```python
from build123d import *

# Parameters (mm, degrees)
SKETCH2_OUTSIDE_W  = 79.82
SKETCH2_OUTSIDE_H  = 79.82
SKETCH2_OUTSIDE_R  = 1.6
CUT_EXTRUDE1_DEPTH = 10
SKETCH3_R          = 12
CUT_EXTRUDE2_DEPTH = 10


with BuildPart() as part:
    # Sketch1 → Revolve1 (revolve)
    with BuildSketch(Plane.XY, mode=Mode.PRIVATE) as revolve1_sk:
        Polygon((0, 0), (0, 13.335), (10.67, 13.335), (10.67, 30), (13.06, 30), (13.06, 14.095), (19.18, 14.095), (19.18, 11.90625), (27.18, 11.90625), (27.18, 0), align=None)
    revolve(revolve1_sk.sketch.rotate(Axis((0, 0, 0), (1, 0, 0)), 90), axis=Axis((0, 0, 0), (1, 0, 0)))  # turned: the seam where the file's is

    # Sketch2 outside → Cut-Extrude1 (cut)
    with BuildSketch(Plane.ZY.offset(-10.67)):
        Rectangle(SKETCH2_OUTSIDE_W, SKETCH2_OUTSIDE_H)
        with BuildLine():
            Line((-14.225, 18.225), (14.225, 18.225))
            ThreePointArc((14.225, 18.225), (17.053427125, 17.053427125), (18.225, 14.225))
            Line((18.225, 14.225), (18.225, -14.225))
            ThreePointArc((18.225, -14.225), (17.053427125, -17.053427125), (14.225, -18.225))
            Line((14.225, -18.225), (-14.225, -18.225))
            ThreePointArc((-14.225, -18.225), (-17.053427125, -17.053427125), (-18.225, -14.225))
            Line((-18.225, -14.225), (-18.225, 14.225))
            ThreePointArc((-18.225, 14.225), (-17.053427125, 17.053427125), (-14.225, 18.225))
        make_face(mode=Mode.SUBTRACT)
        with Locations((-14.29, 14.29)):
            Circle(SKETCH2_OUTSIDE_R)
        with Locations((14.29, 14.29)):
            Circle(SKETCH2_OUTSIDE_R)
        with Locations((14.29, -14.29)):
            Circle(SKETCH2_OUTSIDE_R)
        with Locations((-14.29, -14.29)):
            Circle(SKETCH2_OUTSIDE_R)
    extrude(amount=-CUT_EXTRUDE1_DEPTH, mode=Mode.SUBTRACT)

    # Sketch3 → Cut-Extrude2 (cut)
    with BuildSketch(Plane.ZY):
        Circle(SKETCH3_R)
    extrude(amount=-CUT_EXTRUDE2_DEPTH, mode=Mode.SUBTRACT)


solid = part.part
```
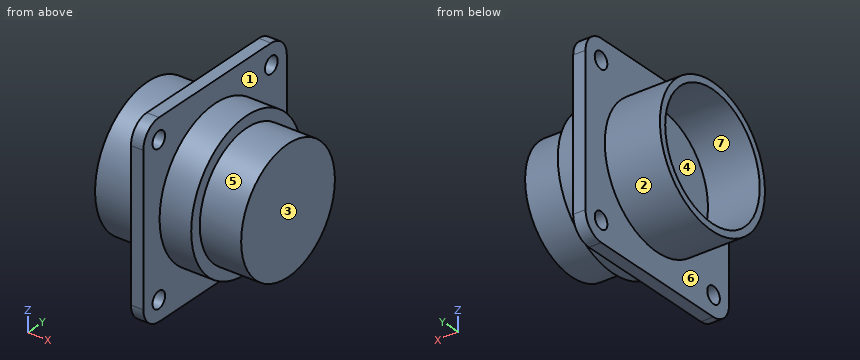
Can you work these out from the model? Positions are in its coordinate system, mm. Face numbers are marked on the shaded views. A direction names the side the tool comes from. Round coordinates to 2 decimals unless told otherwise and drop trailing zeros. Order: outer loops, then holes, each group sorted by start corner. A loop starts at its lowest first (then second) coordinate and runs counter-clockwise, first axis right, second up.
(1) If we section it at D-D (z = 15): Please give me the cut outline in (x, y).
Results are:
outline: (10.67, -18.15) - (13.06, -18.15) - (13.06, -15.72) - (10.67, -15.72) - close; (10.67, -12.86) - (13.06, -12.86) - (13.06, 12.86) - (10.67, 12.86) - close; (10.67, 15.72) - (13.06, 15.72) - (13.06, 18.15) - (10.67, 18.15) - close
(2) I'm going to push flat-ended pins straight in: pin 1 (10 mm diameter, centred on x = 22.5, y = -6.5, fed in from -Z); pin 2 (4 mm diameter, centred on x = 21, z = -3.5, fed in from +Y); pin 3 (3.5 mm diameter, centred on y = 14.29, z = 14.29, fed in from +X); pin 4 (1.9 mm diameter, centred on y = -14.29, z = 14.29, fed in from +X). Where does each tip first touch, or does it pass through?
Results are:
pin 1: stops at z = -13.82
pin 2: stops at y = 13.84
pin 3: stops at x = 13.06
pin 4: passes through
(3) If I drill on L1, parallel to Y at x = 11.8, z = -14.29; L2, parallel to X at y = -10, z = 0.5; L3, parallel to Z at x = 8.25, y = -11, over which ranges is the centre line in solid material (lowest first)?
Results are:
L1: y = -18.22 to -15.89, -12.69 to 12.69, 15.89 to 18.22
L2: x = 10 to 27.18
L3: z = -7.54 to -4.8, 4.8 to 7.54
(4) If we section it at A-A (x = 12.5): Please give me the cut outline in (y, z) (3 decimals).
Results are:
outline: (-18.225, -14.225) arc R4 ccw to (-14.225, -18.225) - (14.225, -18.225) arc R4 ccw to (18.225, -14.225) - (18.225, 14.225) arc R4 ccw to (14.225, 18.225) - (-14.225, 18.225) arc R4 ccw to (-18.225, 14.225) - close; hole circle Ø3.2 at (-14.29, -14.29); hole circle Ø3.2 at (-14.29, 14.29); hole circle Ø3.2 at (14.29, -14.29); hole circle Ø3.2 at (14.29, 14.29)
(5) On a 3-axis mill with a long thin cutter (end or side, diameter ignored), from which of +Z, -Z, +X, -X, +Y, -Y can I reach the whole of each face in a straight line? I mean the marked faces 1, 2 and 3. Say none if no direction works.
Results are:
face 1: +X
face 2: -X
face 3: +Z, -Z, +X, +Y, -Y
(6) We'd pull the mould along Y, two halves only. Please class the marked faces 4, 5, 6 and 7: +Y half, -Y half, draft (parallel to the pull), parting line (faces both ways), or undercut.
Results are:
face 4: undercut
face 5: parting line
face 6: draft
face 7: undercut
(7) If we section it at B-B (y = 0): Please give me the cut outline in (x, z) (3 decimals).
Results are:
outline: (0, -13.335) - (10.67, -13.335) - (10.67, -18.225) - (13.06, -18.225) - (13.06, -14.095) - (19.18, -14.095) - (19.18, -11.906) - (27.18, -11.906) - (27.18, 11.906) - (19.18, 11.906) - (19.18, 14.095) - (13.06, 14.095) - (13.06, 18.225) - (10.67, 18.225) - (10.67, 13.335) - (0, 13.335) - (0, 12) - (10, 12) - (10, -12) - (0, -12) - close
